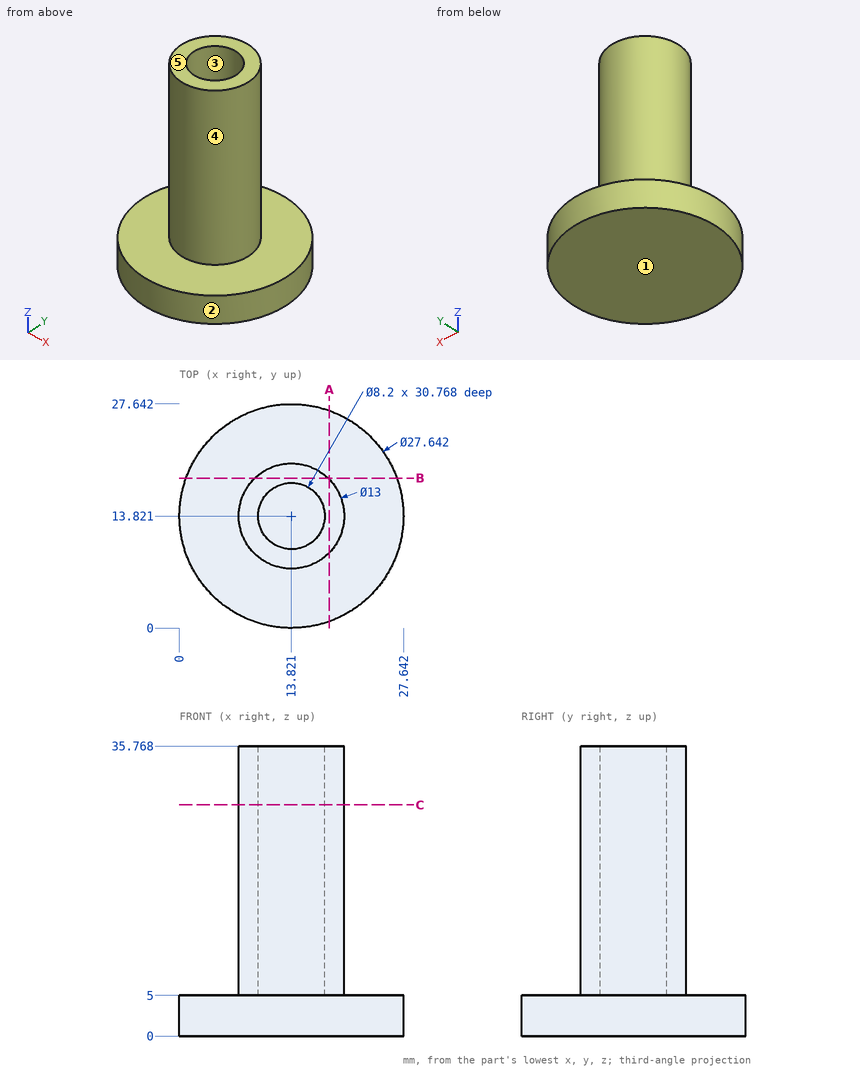
Could you check a few things on this drawing? It's one solid part, dimensions in mm from its lowest x, y, z. A direction names the side the tool comes from. Give positions to 0.01 mm unless a question says otherwise; leave off trailing zeros. Order: outer loops, then holes, each group sorted by start corner. A loop starts at its lowest first (then second) coordinate and runs counter-clockwise, first axis right, second up. Notation, with made-up numbers: M 3,33.5 L 26,33.5 A26 cw 26,50.5 Z; hole C 87,-20.5 d10. An arc over 180 degrees is marked long. Use one line per item in the form item = value. Start each with the question number.
Item 1: If I drill on line 1 along Z through (x, y) = (5.75, 7.5); line 2 along X through (y, z) = (13, 19) (1 decimal); line 3 along X through (y, z) = (12, 8) (1 decimal), over which ranges is the centre line in solid material (lowest first)?
Item 2: Will these pins go through, and if not, where does the flat tip stop? pin 1 Ø1 at (x, y) = (3, 18.5) entering from +Z; pin 2 Ø1 at (y, z) = (8, 27.5) entering from -X; pin 3 Ø3 at (y, z) = (17.5, 30) entering from -X.
Item 3: If we section it at C-C (z = 28.5): Write out the boundary of the cut face in (x, y).
Item 4: If we section it at A-A (x = 18.5): Write out the boundary of the cut face in (y, z) (1 decimal), then the cut area to 3 significant figures.
Item 5: We'd pull the mould along Y, two halves only. Please class the marked faces 1, 2 and 3: +Y half, -Y half, draft (parallel to the pull), parting line (faces both ways), or undercut.
Item 6: For the marked faces 4 and 5, which set-ups out of +Z, -Z, +X, -X, +Y, -Y let a thin tool reach every point of the face, with its end or its side?
Outcome:
q1.line_1 = 0 to 5
q1.line_2 = 7.4 to 9.8, 17.8 to 20.3
q1.line_3 = 7.6 to 10.1, 17.5 to 20.1
q2.pin_1 = 5
q2.pin_2 = 10.09
q2.pin_3 = 7.7
q3.outline = C 13.82,13.82 d13; hole C 13.82,13.82 d8.2
q4.outline = M 0.8,0 L 26.8,0 L 26.8,5 L 18.3,5 L 18.3,35.8 L 9.3,35.8 L 9.3,5 L 0.8,5 Z
q4.area = 408 mm2
q5.face_1 = draft
q5.face_2 = parting line
q5.face_3 = undercut
q6.face_4 = +Z
q6.face_5 = +Z, +X, -X, +Y, -Y
